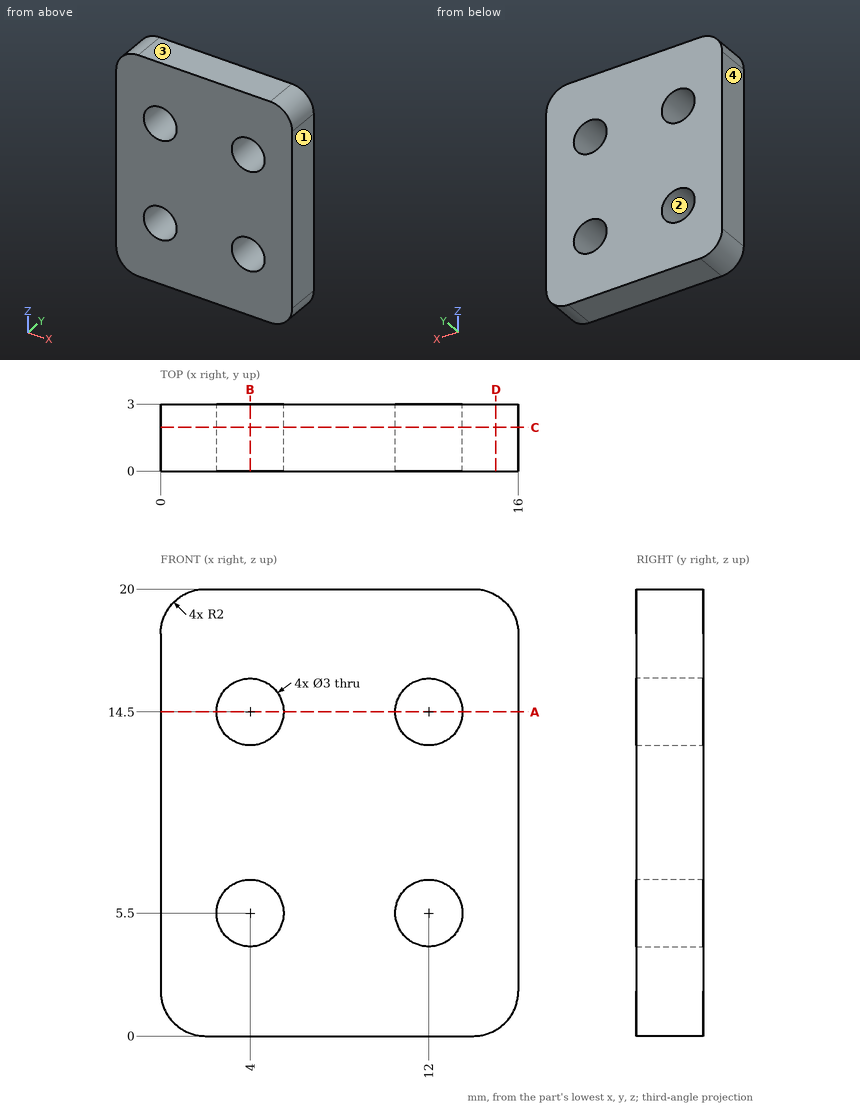
Geometry: see drawing. Coordinates: mm, zero at the bounding-box minimum. Give positions to 0.01 mm unless a question says otherwise; leave off trailing zeros. Write each loop counter-clockwise with the first axis right and the second up, starting at its lowest first coordinate (ties: lowest second). Pieces come first, ordered by that corner, then holes. Notation, with made-up numbers: M 79,66.25 L 126,66.25 A22 ccw 126,79.25 Z; hole C -29.5,19.5 d3. An arc over 180 degrees is marked long. Return JSON: item names as keys, results as strings. Group by question number.
1) Cut plane D-D, the plane x = 15. Output: boundary loops of the cut face in (y, z), then the cut area to 3 significant figures.
2) Cut plane C-C, the plane y = 1.95. Output: boundary loops of the cut face in (x, z), then the cut area to 3 significant figures.
3) First-contact query: pin 1 Ø1.8 at (x, z) = (12, 5.5) entering from +Y. Flat tip, straight axial feed; report the tip coordinate or a pass-through.
4) Cut plane B-B, the plane x = 4. Output: boundary loops of the cut face in (y, z), then the cut area to 3 significant figures.
5) Ray query, L1, parallel to X at y = 1.65, z = 5.5; L2, parallel to Z at x = 13.25, y = 1; L3, parallel to X at y = 1.4, z = 15.75. Return the intervals inside material, ascending.
6) Draft query along X for the marked faces 1, 2, 3 and 4. Return one class per face: released by +X, released by -X, zero draft, split by the parting line, or undercut.
7) Cut plane A-A, the plane z = 14.5. Output: boundary loops of the cut face in (x, y).
Data:
{
 "1": {"outline": "M 0,0.27 L 3,0.27 L 3,19.73 L 0,19.73 Z", "area": "58.4 mm²"},
 "2": {"outline": "M 0,2 A2 ccw 2,0 L 14,0 A2 ccw 16,2 L 16,18 A2 ccw 14,20 L 2,20 A2 ccw 0,18 Z; hole C 4,5.5 d3; hole C 4,14.5 d3; hole C 12,5.5 d3; hole C 12,14.5 d3", "area": "288 mm²"},
 "3": {"pin 1": "passes through"},
 "4": {"outline": "M 0,0 L 3,0 L 3,4 L 0,4 Z; M 0,7 L 3,7 L 3,13 L 0,13 Z; M 0,16 L 3,16 L 3,20 L 0,20 Z", "area": "42.0 mm²"},
 "5": {"L1": "x = 0 to 2.5, 5.5 to 10.5, 13.5 to 16", "L2": "z = 0 to 4.67, 6.33 to 13.67, 15.33 to 20", "L3": "x = 0 to 3.17, 4.83 to 11.17, 12.83 to 16"},
 "6": {"face 1": "released by +X", "face 2": "undercut", "face 3": "zero draft", "face 4": "released by -X"},
 "7": {"outline": "M 0,0 L 2.5,0 L 2.5,3 L 0,3 Z; M 5.5,0 L 10.5,0 L 10.5,3 L 5.5,3 Z; M 13.5,0 L 16,0 L 16,3 L 13.5,3 Z"}
}
